from build123d import *

# Parameters (mm, degrees)
SKETCH1_R           = 8.977796406
TOOTHOD_DEPTH       = 7.9375
TOOTHPROFILE_DEPTH  = 16.875
TOOTHPATTERN_COUNT  = 12
SKETCH7_R           = 4
BORE_DEPTH          = 10.2075
BORE_DEPTH_BACK     = 10.2075
BOSS_EXTRUDE1_START = -2.54
BOSS_EXTRUDE1_DEPTH = 15.875


with BuildPart() as part:
    # Sketch1 → ToothOD (new body, symmetric)
    with BuildSketch(Plane(origin=(0, 0, 0), x_dir=(1, 0, 0), z_dir=(0, 1, 0))):
        Circle(SKETCH1_R)
    extrude(amount=TOOTHOD_DEPTH, both=True)

    # Sketch2 → ToothProfile (cut, through all)
    with BuildSketch(Plane(origin=(0, 7.9375, 0), x_dir=(1, 0, 0), z_dir=(0, 1, 0))):
        with BuildLine():
            ThreePointArc((-1.501752794, 8.177535128), (0, 6.917796406), (1.501752794, 8.177535128))
            ThreePointArc((1.501752794, 8.177535128), (1.784898523, 8.602004268), (2.28897191, 8.681096469))
            ThreePointArc((2.28897191, 8.681096469), (0, 8.977796406), (-2.28897191, 8.681096469))
            ThreePointArc((-2.28897191, 8.681096469), (-1.784898523, 8.602004268), (-1.501752794, 8.177535128))
        make_face()
    toothprofile = extrude(amount=-TOOTHPROFILE_DEPTH, mode=Mode.SUBTRACT)

    # ToothPattern: ToothProfile ×12 about axis
    toothpattern_axis = Axis((0, 0, 0), (0, 1, 0))
    for i in range(1, TOOTHPATTERN_COUNT):
        add(toothprofile.rotate(toothpattern_axis, i * 360 / TOOTHPATTERN_COUNT), mode=Mode.SUBTRACT)

    # Sketch4 → Flange (revolve)
    with BuildSketch(Plane.XY):
        with BuildLine():
            Line((0, -7.9375), (9.231796406, -7.9375))
            ThreePointArc((9.231796406, -7.9375), (9.557552396, -7.963122571), (9.877368734, -8.030137424))
            ThreePointArc((9.877368734, -8.030137424), (10.445097311, -8.311697125), (10.946296406, -8.6995))
            Line((10.946296406, -8.6995), (10.946296406, -9.2075))
            Line((10.946296406, -9.2075), (0, -9.2075))
            Line((0, -9.2075), (0, -7.9375))
        make_face()
        with BuildLine():
            Line((10.946296406, 9.2075), (10.946296406, 8.6995))
            ThreePointArc((10.946296406, 8.6995), (10.445097311, 8.311697125), (9.877368734, 8.030137424))
            ThreePointArc((9.877368734, 8.030137424), (9.557552396, 7.963122571), (9.231796406, 7.9375))
            Line((9.231796406, 7.9375), (0, 7.9375))
            Line((0, 7.9375), (0, 9.2075))
            Line((0, 9.2075), (10.946296406, 9.2075))
        make_face()
    revolve(axis=Axis((0, 12.09802, 0), (0, -1, 0)))

    # Sketch7 → Bore (cut, two sides)
    with BuildSketch(Plane.XZ) as bore_sk:
        Circle(SKETCH7_R)
    extrude(amount=BORE_DEPTH, mode=Mode.SUBTRACT)
    extrude(bore_sk.sketch, amount=-BORE_DEPTH_BACK, mode=Mode.SUBTRACT)

    # Sketch8 → Boss-Extrude1 (add, through all)
    with BuildSketch(Plane.XZ.offset(9.2075).offset(BOSS_EXTRUDE1_START)):
        with BuildLine():
            Line((-2.645751311, 3), (2.645751311, 3))
            ThreePointArc((2.645751311, 3), (0, 4), (-2.645751311, 3))
        make_face()
    extrude(amount=-BOSS_EXTRUDE1_DEPTH)


solid = part.part
Work out the finished part from the listing and answer in its coordinate system (mm). A direction names the side the tool comes from. Coordinates: 2 decimals unless noted, no trailing zeros. Loops run counter-clockwise (first coordinate to the right, second up) from the corner with the lowest first, then second, coordinate; pieces in that order, holes last. Notation, with made-up numbers: M -12.5,-5.75 L 36.5,-5.75 A19 ccw 36.5,18.25 Z; hole C -29.5,-1.75 d7. An arc over 180 degrees is marked long. Answer in a Markdown table with one row per item. Add a question column.
1. The mould has two halves that part along Z. Classify faces 1 (the flat face through (0, 1, 3)), 2 (the cylindrical face through (-0.03, 0.11, -6.92)), 3 (the cylindrical face through (10.44, 8.95, 3.29)), 4 (the cylindrical face through (-2.759, 0.111, -8.335)): pulls with the +Z half, pulls with the -Z half, needs draft (parallel to the pull), parting line crosses it, or undercut.
2. Find section B-B, the plane x = 0. Write down the section's boundary in (y, z).
3. Flat-ended cylindrical pins translate along their axes: P1, Ø3, axis at x = 2, y = 6, coming from the -Z side; P2, Ø2.5, axis at x = 0.5, y = 4.5, coming from the -Z side; P3, Ø3, axis at y = 0, z = -6.5, coming from the +X side. Find the tip coordinate at first contact, or state that the pin passes through.
4. Consider L1, parallel to Z at x = -6.25, y = -6; L2, parallel to Z at x = 0, y = -2.5; L3, parallel to Y at x = -8, z = 0.25. Determine where each line is inside the solid, lowest interval first.
5. A tool of negligible diameter and unlimited length cuts with its end or side. For faces 5 (the cylindrical face through (-6.557, 0.111, 5.854)), 6 (the cylindrical face through (5.839, 0.111, -6.557)), 7 (the cylindrical face through (-5.839, 0.111, 6.557)), 8 (the flat face through (-4, -7.937, -6)), 9 (the flat face through (0, -6.667, 3.4)), from which of +Z, -Z, +X, -X, +Y, -Y can it reach the whole face along a straight path? Write none if from no direction.
6. Find section A-A, the plane z = 0. Write down the section's boundary in (x, y), then the cut area to 3 significant figures.
Reported:
| question | item | result |
|---|---|---|
| 1 | face 1 | undercut |
| 1 | face 2 | pulls with the -Z half |
| 1 | face 3 | parting line crosses it |
| 1 | face 4 | undercut |
| 2 | outline | M -9.21,-10.95 L -8.7,-10.95 A3.2 ccw -8.03,-9.88 A2.55 ccw -7.94,-9.23 L -7.94,-6.92 L 7.94,-6.92 L 7.94,-9.23 A2.55 ccw 8.03,-9.88 A3.2 ccw 8.7,-10.95 L 9.21,-10.95 L 9.21,-4 L -9.21,-4 Z; M -9.21,4 L -6.67,4 L -6.67,3 L 9.21,3 L 9.21,10.95 L 8.7,10.95 A3.2 ccw 8.03,9.88 A2.55 ccw 7.94,9.23 L 7.94,6.92 L -7.94,6.92 L -7.94,9.23 A2.55 ccw -8.03,9.88 A3.2 ccw -8.7,10.95 L -9.21,10.95 Z |
| 3 | P1 | stops at z = -8.7 |
| 3 | P2 | stops at z = -8.58 |
| 3 | P3 | stops at x = 6.56 |
| 4 | L1 | z = -6.44 to -5.32, -3.13 to 3.13, 5.32 to 6.44 |
| 4 | L2 | z = -6.92 to -4, 3 to 6.92 |
| 4 | L3 | y = -9.21 to -7.94, 7.94 to 9.21 |
| 5 | face 5 | -X |
| 5 | face 6 | -Z |
| 5 | face 7 | +Z |
| 5 | face 8 | none |
| 5 | face 9 | -Y |
| 6 | outline | M -10.95,-9.21 L -4,-9.21 L -4,9.21 L -10.95,9.21 L -10.95,8.7 A3.2 ccw -9.88,8.03 A2.55 ccw -9.23,7.94 L -6.92,7.94 L -6.92,-7.94 L -9.23,-7.94 A2.55 ccw -9.88,-8.03 A3.2 ccw -10.95,-8.7 Z; M 4,-9.21 L 10.95,-9.21 L 10.95,-8.7 A3.2 ccw 9.88,-8.03 A2.55 ccw 9.23,-7.94 L 6.92,-7.94 L 6.92,7.94 L 9.23,7.94 A2.55 ccw 9.88,8.03 A3.2 ccw 10.95,8.7 L 10.95,9.21 L 4,9.21 Z |
| 6 | area | 126 mm^2 |
